Could you check a few things on this drawing? It's one solid part, dimensions in mm from its lowest x, y, z. A direction names the side the tool comes from. Round coordinates to 2 decimals unless told otherwise and drop trailing zeros. Loops run counter-clockwise (first coordinate to the right, second up) from the corner with the lowest first, then second, coordinate; pieces in that order, holes last. Notation, with made-up numbers: M 89.25,49.5 L 123.25,49.5 A20 ccw 123.25,68.5 Z; hole C 65,6 d4. An arc over 180 degrees is marked long. Answer as a JSON object with one key per item and string values.
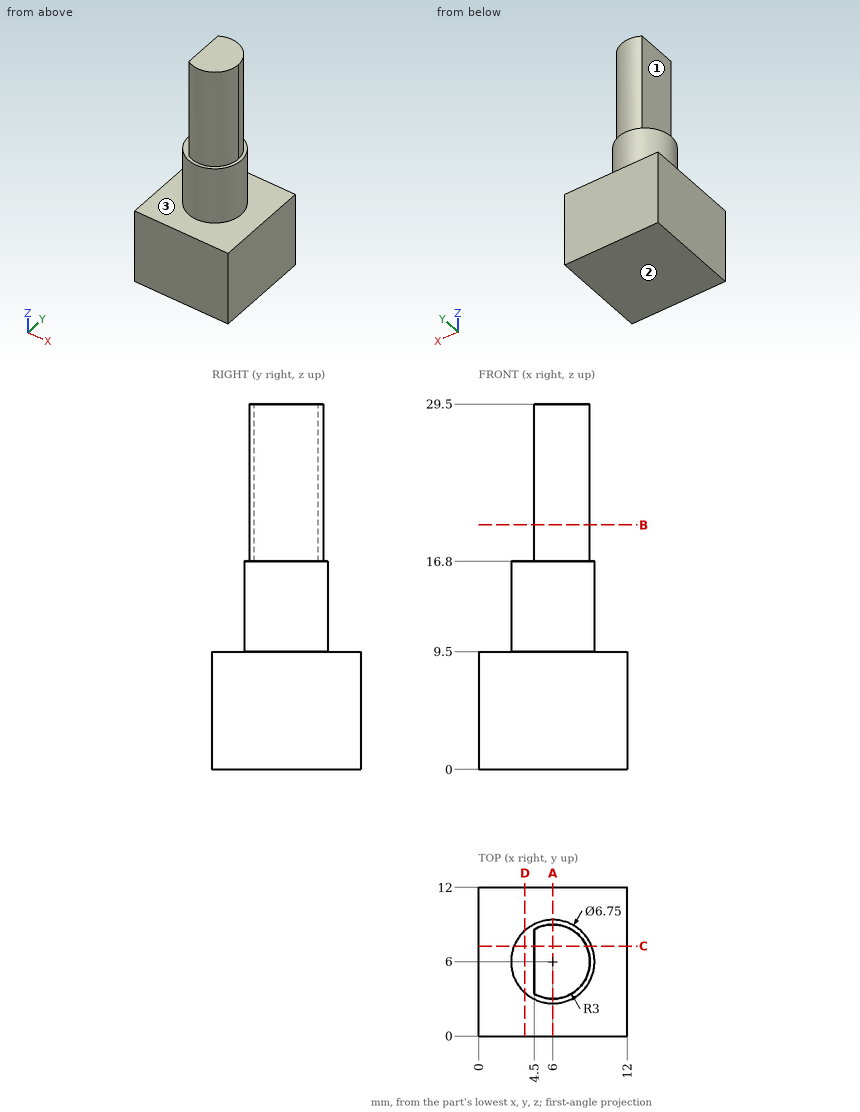
Item 1: I want a section at D-D, the plane x = 3.75. Please give me the cut outline in (y, z), then the cut area to 3 significant figures.
Resolved:
{"outline": "M 0,0 L 12,0 L 12,9.5 L 8.52,9.5 L 8.52,16.8 L 3.48,16.8 L 3.48,9.5 L 0,9.5 Z", "area": "151 mm²"}
Item 2: I want a section at C-C, the plane y = 7.25. Please give me the cut outline in (x, z).
Resolved:
{"outline": "M 0,0 L 12,0 L 12,9.5 L 9.13,9.5 L 9.13,16.8 L 8.73,16.8 L 8.73,29.5 L 4.5,29.5 L 4.5,16.8 L 2.87,16.8 L 2.87,9.5 L 0,9.5 Z"}
Item 3: Please list where these lines run through material, in increasing order: probe 1 along X at (y, z) = (4.5, 27.25); probe 2 along Z at (x, y) = (0.75, 8.25); probe 3 along X at (y, z) = (3, 14). Write a range as from..to.
Resolved:
{"probe 1": "4.5..8.6", "probe 2": "0..9.5", "probe 3": "4.45..7.55"}
Item 4: I want a section at B-B, the plane z = 19.75. Please give me the cut outline in (x, y), then the cut area to 3 significant figures.
Resolved:
{"outline": "M 4.5,3.4 A3 ccw long 4.5,8.6 Z", "area": "22.7 mm²"}
Item 5: On a 3-axis mill with a long thin cutter (end or side, diameter ignored), from which of +Z, -Z, +X, -X, +Y, -Y can I reach the whole of each face in a straight line? I mean the marked faces 1, 2 and 3. Say none if no direction works.
Resolved:
{"face 1": "+Z, -X, +Y, -Y", "face 2": "-Z, +X, -X, +Y, -Y", "face 3": "+Z"}
Item 6: I want a section at A-A, the plane x = 6. Please give me the cut outline in (y, z) (3 decimals), then the cut area to 3 significant figures.
Resolved:
{"outline": "M 0,0 L 12,0 L 12,9.5 L 9.375,9.5 L 9.375,16.8 L 9,16.8 L 9,29.5 L 3,29.5 L 3,16.8 L 2.625,16.8 L 2.625,9.5 L 0,9.5 Z", "area": "239 mm²"}
Item 7: I'm going to push flat-ended pins straight in: pin 1 Ø2.5 at (y, z) = (5.5, 24.5) entering from -X; pin 2 Ø5 at (x, z) = (10.5, 14) entering from +Y. Where does each tip first touch, or does it pass through?
Resolved:
{"pin 1": "x = 4.5", "pin 2": "y = 8.72"}
